Geometry: final body of the model. Coordinates: model frame, mm. Give positions to 0.01 mm unless a question says otherwise; leave off trailing zeros. Write each loop counter-clockwise with the first axis right and the second up, starting at its lowest first coordinate (ties: lowest second). Pieces come first, ordered by that corner, then holes. Notation, with made-up numbers: (71, 36.25) -> (119, 36.25) arc R12 cw to (119, 40.25) -> close; hole circle Ø7 at (-8.5, 4). An arc over 180 degrees is marked (long way). Answer as a JSON object with one key per item and string values. Group by question number.
(1) Material intervals for probe 1 along Z at (x, y) = (3.5, 8.75) (3 decimals); probe 2 along Y at (x, z) = (-0.25, 427); probe 3 along Y at (x, z) = (-1.25, 376.5), sorted ascending.
(2) Section query A-A on x = 0. Output: boundary loops of the cut face in (y, z) (3 decimals), plus the area to 3 significant figures.
(3) Section query C-C on z = 157.5. Output: boundary loops of the cut face in (x, y) (3 decimals).
(4) Contact query for flat-ended pins moving along their axis: pin 1 Ø1 at (x, z) = (-2.5, 455.5) entering from -Y; pin 2 Ø6 at (y, z) = (-7.5, 86) entering from -X (3 decimals); pin 3 Ø6 at (x, z) = (-5.5, 471) entering from +Y; pin 4 Ø4 at (x, y) = (-6.5, 1.5) entering from -Z. Output: stop coordinate, or through.
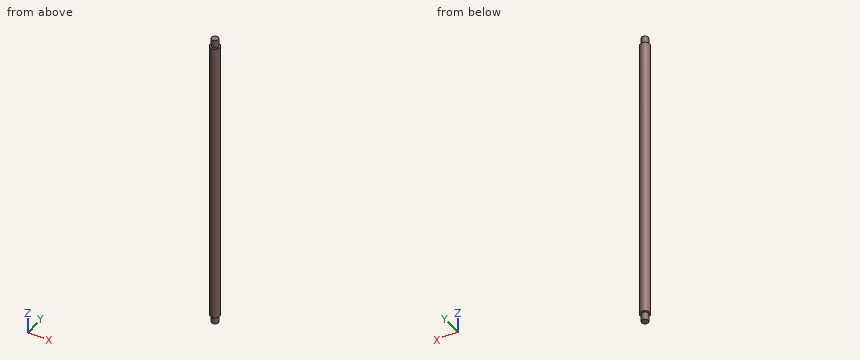
from build123d import *

# Parameters (mm, degrees)
BOSS_EXTRUDE3_DEPTH      = 596.9
BOSS_EXTRUDE3_DEPTH_BACK = 12.7
SKETCH1_R                = 6.35
BOSS_EXTRUDE4_START      = 3.175
SKETCH3_R                = 9.525
BOSS_EXTRUDE4_DEPTH      = 577.85


with BuildPart() as part:
    # Sketch1 → Boss-Extrude3 (new, two sides: drawn at the far end of the back side and taken through both)
    with BuildSketch(Plane.XY.offset(-BOSS_EXTRUDE3_DEPTH_BACK)):
        with Locations(Location((0, 0, 0), (0, 0, 270))):
            Circle(SKETCH1_R)
    extrude(amount=BOSS_EXTRUDE3_DEPTH + BOSS_EXTRUDE3_DEPTH_BACK)

    # Sketch3 → Boss-Extrude4 (add)
    with BuildSketch(Plane.XY.offset(BOSS_EXTRUDE4_START)):
        with Locations(Location((0, 0, 0), (0, 0, 180))):
            Circle(SKETCH3_R)
    extrude(amount=BOSS_EXTRUDE4_DEPTH)


solid = part.part
Answer list:
{
 "1": {"probe 1": "3.175 to 581.025", "probe 2": "-9.52 to 9.52", "probe 3": "-9.44 to 9.44"},
 "2": {"outline": "(-9.525, 3.175) -> (-6.35, 3.175) -> (-6.35, -12.7) -> (6.35, -12.7) -> (6.35, 3.175) -> (9.525, 3.175) -> (9.525, 581.025) -> (6.35, 581.025) -> (6.35, 596.9) -> (-6.35, 596.9) -> (-6.35, 581.025) -> (-9.525, 581.025) -> close", "area": "11,400 mm2"},
 "3": {"outline": "circle Ø19.05 at (0, 0)"},
 "4": {"pin 1": "y = -9.31", "pin 2": "x = -8.395", "pin 3": "y = 9.19", "pin 4": "z = -12.7"}
}
